Could you check a few things on this model? Use its own coordinates, in mm. A direction names the side the tool comes from. Give positions to 0.01 mm unless a question says otherwise; leave off trailing zeros. Write each loop counter-clockwise with the first axis right and the second up, starting at its lowest first coordinate (ties: lowest second). Pieces come first, ordered by that corner, then holes. Notation, with made-up numbers: M -25,-13.75 L 14,-13.75 A17 ccw 14,6.25 Z; hole C 31,-6 d7. An arc over 180 degrees is marked long. Answer as CSV lines item,"result". Start each with the question number.
from build123d import *

# Parameters (mm, degrees)
SKETCH5_OUTSIDE_W   = 34.468
SKETCH5_OUTSIDE_H   = 34.468
CUT_EXTRUDE1_DEPTH  = 7.2
BOSS_EXTRUDE1_REACH = 51.718
SKETCH10_R          = 10.705
SKETCH10_R_2        = 6.9
BOSS_EXTRUDE3_REACH = 31.655
SKETCH12_R          = 8.3
CUT_EXTRUDE3_REACH  = 52.072
SKETCH13_R          = 4.25
CUT_EXTRUDE4_DEPTH  = 18.944444
CUT_EXTRUDE5_START  = -25.5
SKETCH19_R          = 5.15
CUT_EXTRUDE5_DEPTH  = 25.5
CUT_EXTRUDE6_START  = -43.255556
SKETCH20_R          = 28.536151212
CUT_EXTRUDE6_DEPTH  = 43.255556
SKETCH22_R          = 6.55
SKETCH22_R_2        = 5.15
SKETCH23_R          = 5.15
BOSS_EXTRUDE4_DEPTH = 3


# Read off the part's stored shape, not the designer's step: Cut-Extrude2
with BuildPart() as part:
    # Sketch1 → Revolve1 (revolve)
    with BuildSketch(Plane.XY, mode=Mode.PRIVATE) as revolve1_sk:
        Polygon((3.25, 47.7), (6.15, 47.7), (6.55, 43.217813034), (6.15, 42.533333333), (6.55, 38.051146367), (6.15, 37.366666667), (6.55, 32.8844797), (6.15, 32.2), (6.55, 26.2), (6.55, 22.2), (10.6, 22.2), (10.6, 15), (8.3, 15), (8.3, 0), (5.5, 0), (5.5, 18), (3.25, 19.7), align=None)
    revolve(revolve1_sk.sketch.rotate(Axis((0, 0, 0), (0, 1, 0)), 90), axis=Axis((0, 0, 0), (0, 1, 0)))

    # Sketch5 outside → Cut-Extrude1 (cut)
    with BuildSketch(Plane(origin=(0, 22.2, 0), x_dir=(1, 0, 0), z_dir=(0, 1, 0))):
        Rectangle(SKETCH5_OUTSIDE_W, SKETCH5_OUTSIDE_H)
        Polygon((-5.3, 9.17986928), (5.3, 9.17986928), (10.6, 0), (5.3, -9.17986928), (-5.3, -9.17986928), (-10.6, 0), align=None, mode=Mode.SUBTRACT)
    extrude(amount=-CUT_EXTRUDE1_DEPTH, mode=Mode.SUBTRACT)

    # Sketch4 → Cut-Revolve1 (revolve, cut)
    with BuildSketch(Plane.XY, mode=Mode.PRIVATE) as cut_revolve1_sk:
        Polygon((6.9, 0), (8.3, 1.4), (8.3, 0), align=None)
        Polygon((8.3, 15), (10.6, 15.837131539), (10.6, 15), align=None)
        Polygon((8.3, 22.2), (10.6, 21.362868461), (10.6, 22.2), align=None)
    revolve(cut_revolve1_sk.sketch.rotate(Axis((0, 0, 0), (0, 1, 0)), 90), axis=Axis((0, 0, 0), (0, 1, 0)), mode=Mode.SUBTRACT)

    # Boss-Extrude1: up to this cone (the profile starts outside it)
    boss_extrude1_end = Plane(origin=(0, 0, 0), z_dir=(0, 1, 0)).offset(11.979048056) * Cone(2.747e-06, 110.555614597, 40.238951944, align=(Align.CENTER, Align.CENTER, Align.MIN), mode=Mode.PRIVATE)
    # Sketch10 → Boss-Extrude1 (add, up to the surface)
    with BuildSketch(Plane.XZ, mode=Mode.PRIVATE) as boss_extrude1_sk1:
        with Locations(Location((0, 0, 0), (0, 0, 270))):
            Circle(SKETCH10_R)
        Circle(SKETCH10_R_2, mode=Mode.SUBTRACT)
    boss_extrude1_tool1 = extrude(boss_extrude1_sk1.sketch, amount=-BOSS_EXTRUDE1_REACH, mode=Mode.PRIVATE) - boss_extrude1_end
    add(boss_extrude1_tool1.solids().sort_by_distance((0, 0, 10.402217))[0])

    # Cut-Extrude2 outline → Cut-Extrude2 (revolve, cut)
    with BuildSketch(Plane.XY):
        Polygon((7.874, 16.206311111), (5.5, 18), (5.5, 0), (7.874, 0), align=None)
    revolve(axis=Axis((0, 0, 0), (0, 1, 0)), mode=Mode.SUBTRACT)

    # Boss-Extrude3: up to this cone (the profile starts inside it)
    boss_extrude3_end = Plane(origin=(0, 22.2, 0), z_dir=(0, 1, 0)).offset(-10.220951944) * Cone(2.747e-06, 193.581188051, 70.457789364, align=(Align.CENTER, Align.CENTER, Align.MIN), mode=Mode.PRIVATE)
    # Sketch12 → Boss-Extrude3 (add, up to the surface)
    with BuildSketch(Plane(origin=(0, 22.2, 0), x_dir=(1, 0, 0), z_dir=(0, 1, 0)), mode=Mode.PRIVATE) as boss_extrude3_sk1:
        Polygon((-5.415470054, 9.37986928), (-10.830940108, 0), (-5.415470054, -9.37986928), (5.415470054, -9.37986928), (10.830940108, 0), (5.415470054, 9.37986928), align=None)
        Circle(SKETCH12_R, mode=Mode.SUBTRACT)
    boss_extrude3_tool1 = extrude(boss_extrude3_sk1.sketch, amount=-BOSS_EXTRUDE3_REACH, mode=Mode.PRIVATE) & boss_extrude3_end
    add(boss_extrude3_tool1.solids().sort_by_distance((-7.875037, 22.2, -4.546655))[0])

    # Cut-Extrude3: up to this cone (the profile starts outside it)
    cut_extrude3_end = Plane(origin=(0, 47.7, 0), z_dir=(0, -1, 0)).offset(25.544445444) * Cone(1.324e-06, 35.771764706, 27.027554556, align=(Align.CENTER, Align.CENTER, Align.MIN), mode=Mode.PRIVATE)
    # Sketch13 → Cut-Extrude3 (cut, up to the surface)
    with BuildSketch(Plane(origin=(0, 47.7, 0), x_dir=(1, 0, 0), z_dir=(0, 1, 0)), mode=Mode.PRIVATE) as cut_extrude3_sk1:
        with Locations(Location((0, 0, 0), (0, 0, 270))):
            Circle(SKETCH13_R)
    cut_extrude3_tool1 = extrude(cut_extrude3_sk1.sketch, amount=-CUT_EXTRUDE3_REACH, mode=Mode.PRIVATE) - cut_extrude3_end
    add(cut_extrude3_tool1.solids().sort_by_distance((0, 47.7, 0))[0], mode=Mode.SUBTRACT)

    # Sketch15 → Cut-Extrude4 (cut)
    with BuildSketch(Plane(origin=(0, 18.944444444, 0), x_dir=(-1, 0, 0), z_dir=(0, -1, 0))):
        Polygon((11.188972746, 19.37986928), (-11.188972746, 19.37986928), (-22.377945491, 0), (-11.188972746, -19.37986928), (11.188972746, -19.37986928), (22.377945491, 0), align=None)
    extrude(amount=CUT_EXTRUDE4_DEPTH, mode=Mode.SUBTRACT)

    # Sketch18 → Revolve2 (revolve)
    with BuildSketch(Plane(origin=(0, 0, 0), x_dir=(0, 0, -1), z_dir=(1, 0, 0))):
        Polygon((4.25, 18.944444444), (3.551797403, -21.055555556), (4.551797403, -21.055555556), (5.25, 18.944444444), align=None)
    revolve(axis=Axis((0, 18.944444444, 0), (0, 1, 0)))

    # Sketch19 → Cut-Extrude5 (cut)
    with BuildSketch(Plane(origin=(0, 47.7, 0), x_dir=(1, 0, 0), z_dir=(0, 1, 0)).offset(CUT_EXTRUDE5_START)):
        with Locations(Location((0, 0, 0), (0, 0, 270))):
            Circle(SKETCH19_R)
    extrude(amount=CUT_EXTRUDE5_DEPTH, mode=Mode.SUBTRACT)

    # Sketch20 → Cut-Extrude6 (cut)
    with BuildSketch(Plane.XZ.offset(21.055555556).offset(CUT_EXTRUDE6_START)):
        Circle(SKETCH20_R)
    extrude(amount=CUT_EXTRUDE6_DEPTH, mode=Mode.SUBTRACT)

    # Sweep2: sweep along a path in Sketch21
    with BuildLine(Plane(origin=(0, 0, 0), x_dir=(0, 0, -1), z_dir=(1, 0, 0))) as sweep2_path:
        Line((0, 22.2), (0, 20.2))
        ThreePointArc((0, 20.2), (1.621535411, 12.04799099), (6.239277577, 5.137051454))
    # Sketch22 → Sweep2 (sweep)
    with BuildSketch(Plane.XZ.offset(-22.2)):
        Circle(SKETCH22_R)
        Circle(SKETCH22_R_2, mode=Mode.SUBTRACT)
    sweep(path=sweep2_path.line)

    # Sketch23 → Boss-Extrude4 (add)
    with BuildSketch(Plane(origin=(0, -0.551113062, -0.551113062), x_dir=(1, 0, 0), z_dir=(0, -0.7071067811865513, -0.7071067811865437))):
        Polygon((9.706986403, -13.21553795), (9.331934473, -2.223411857), (-0.37505193, 2.947846691), (-9.706986403, -2.873020855), (-9.331934473, -13.865146949), (0.37505193, -19.036405496), align=None)
        with Locations(Location((0, -8.044279403, 0), (0, 0, 90))):
            Circle(SKETCH23_R, mode=Mode.SUBTRACT)
    extrude(amount=BOSS_EXTRUDE4_DEPTH)

    # Sketch26 → Revolve3 (revolve)
    with BuildSketch(Plane(origin=(-3.338098244, 4.430699396, -4.430699396), x_dir=(0.8825718445701068, 0.33246574197360307, -0.3324657419736067), z_dir=(0.47017756132350597, -0.6240725361798388, 0.6240725361798455)), mode=Mode.PRIVATE) as revolve3_sk:
        Polygon((10.932239672, -3.779391566), (10.282239672, -43.779391566), (8.282239672, -43.779391566), (8.932239672, -3.779391566), align=None)
    revolve(revolve3_sk.sketch.rotate(Axis((0, -0.625868813, -12.002197844), (0, 0.7071067811865513, 0.7071067811865438)), 61.954176959), axis=Axis((0, -0.625868813, -12.002197844), (0, 0.7071067811865513, 0.7071067811865438)))


solid = part.part
1. Please list where these lines run through material, in increasing order: line 1 (Z direction, x = 0, y = 21.2); line 2 (X direction, y = 27.5, z = 4.5).
2. Imagine slicing it at B-B, the plane z = -15. State how many separate pieces and enclosed holes the cut face has, plus the area to 3 significant figures.
3. Will these pins go through, and if not, where does the flat tip stop? P1, Ø4, axis at y = 22, z = -3.5, coming from the +X side; P2, Ø6, axis at x = 0, z = 0, coming from the -Y side; P3, Ø4, axis at y = -20.5, z = -31, coming from the -X side.
4. On a 3-axis mill with a long thin cutter (end or side, diameter ignored), from which of +Z, -Z, +X, -X, +Y, -Y can I reach the whole of each face in a straight line? I mean faces 4 (the conical face through (-1.89, 35.59, -6.02)), 5 (the flat face through (-4.98, -1.65, -1.54)). Say none if no direction works.
5. Thinking about a two-plate mould opening in Z: for faces 1 (the cylindrical face through (3.134, 6.981, -10.175)), 2 (the flat face through (4, 47.7, -4)), 3 (the conical face through (-1.89, 40.76, -6.02)), which applies, pulls with the +Z half, pulls with the -Z half, needs draft (parallel to the pull), parting line crosses it, or undercut?
6. Imagine slicing it at A-A, the plane y = 28.5. Please give me the cut outline in (x, z), plus the area to 3 significant figures.
Solutions:
1,line 1,"-6.55 to -5.15, 5.15 to 6.55"
1,line 2,"-4.64 to -2.5, 2.5 to 4.64"
2,separate pieces,"2"
2,enclosed holes,"1"
2,area,"113 mm²"
3,P1,"x = 6.38"
3,P2,"y = -4.76"
3,P3,"x = -6.65"
4,face 4,"none"
4,face 5,"+Z, -X, -Y"
5,face 1,"undercut"
5,face 2,"needs draft"
5,face 3,"parting line crosses it"
6,outline,"C 0,0 d12.79; hole C 0,0 d10.3"
6,area,"45.2 mm²"
